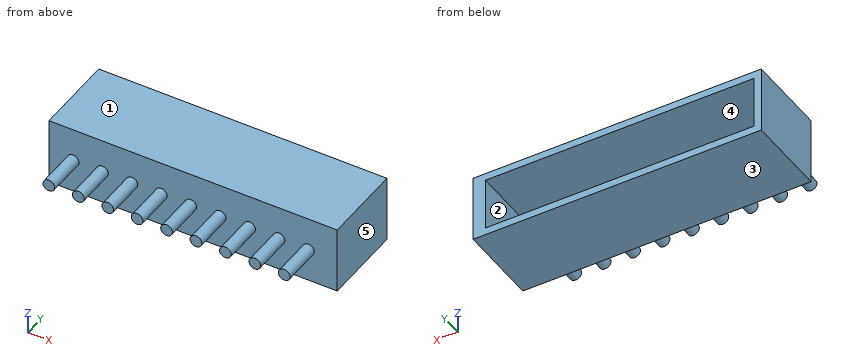
from build123d import *

# Parameters (mm, degrees)
F0_W     = 24.5
F0_H     = 5.7
F1_DEPTH = 7
F2_R     = 0.5
F3_DEPTH = 3.4
F4_W     = 22.82576
F4_H     = 4.464458
F5_DEPTH = 6.35


with BuildPart() as f1:
    # F0 (on Front) → F1 (new body)
    with BuildSketch(Plane.XZ):
        Rectangle(F0_W, F0_H)
    extrude(amount=F1_DEPTH)

    # F2 (on face) → F3 (join)
    with BuildSketch(Plane.XZ.offset(7)):
        with Locations((9.8, 0)):
            Circle(F2_R)
        with Locations((7.3, 0)):
            Circle(F2_R)
        with Locations((4.8, 0)):
            Circle(F2_R)
        with Locations((2.3, 0)):
            Circle(F2_R)
        with Locations((-0.2, 0)):
            Circle(F2_R)
        with Locations((-2.7, 0)):
            Circle(F2_R)
        with Locations((-5.2, 0)):
            Circle(F2_R)
        with Locations((-7.7, 0)):
            Circle(F2_R)
        with Locations((-10.2, 0)):
            Circle(F2_R)
    extrude(amount=F3_DEPTH)

    # F4 (on face) → F5 (cut)
    with BuildSketch(Plane(origin=(0, 0, 0), x_dir=(-1, 0, 0), z_dir=(0, 1, 0))):
        with Locations((0.214789, 0)):
            Rectangle(F4_W, F4_H)
    extrude(amount=-F5_DEPTH, mode=Mode.SUBTRACT)


solid = f1.part
Design review of the part built by this model. Coordinates are the model's own, in mm. Face numbers are marked on the shaded views. A direction names the side the tool comes from. Round coordinates to 2 decimals unless told otherwise and drop trailing zeros. Write each loop counter-clockwise with the first axis right and the second up, starting at its lowest first coordinate (ties: lowest second). Pieces come first, ordered by that corner, then holes. Notation, with made-up numbers: (-35.75, 84) - (-29.75, 84) arc R15 cw to (-29.75, 94) - close; hole circle Ø3 at (32.25, 27.25). An arc over 180 degrees is marked (long way). Return JSON: item names as keys, results as strings. Group by question number.
Item 1: We need section A-A on y = -9.5. Give the number of separate pieces and of enclosed holes in the cut face, and give its area (3 significant figures).
Item 2: Machinability: for the marked faces 1 and 2, which of the approach directions +Z, -Z, +X, -X, +Y, -Y give a long, thin tool a straight path to every point of the face, cutting with its end or side? Answer none if there is none.
Item 3: For probe 1 along X at (y, z) = (-5.75, 1.35); probe 2 along Z at (x, y) = (10.25, -5.75); probe 3 along Y at (x, z) = (-6, -1.8), list the stretches that pass through material, from the lowest coordinate up. Write a range as [from, to].
Item 4: The part is to be moulded in two halves that separate along X. For the marked faces 3, 4 and 5, say which applies: pulls with the +X half, pulls with the -X half, needs draft (parallel to the pull), parting line crosses it, or undercut.
Item 5: We need section D-D on z = -0.8. Write out the cut boundary in (x, y), and give its area (3 significant figures).
Item 6: We need section B-B on y = -4.5. Write out the cut boundary in (x, z).
Item 7: We need section C-C on x = 4.8. Write out the cut boundary in (y, z).
Model answer:
{
 "1": {"separate pieces": "9", "enclosed holes": "0", "area": "7.07 mm²"},
 "2": {"face 1": "+Z, +X, -X, +Y, -Y", "face 2": "+Y"},
 "3": {"probe 1": "x = [-12.25, -11.63], [11.2, 12.25]", "probe 2": "z = [-2.85, -2.23], [2.23, 2.85]", "probe 3": "y = [-7, -6.35]"},
 "4": {"face 3": "needs draft", "face 4": "undercut", "face 5": "pulls with the +X half"},
 "5": {"outline": "(-12.25, -7) - (12.25, -7) - (12.25, 0) - (11.2, 0) - (11.2, -6.35) - (-11.63, -6.35) - (-11.63, 0) - (-12.25, 0) - close", "area": "26.6 mm²"},
 "6": {"outline": "(-12.25, -2.85) - (12.25, -2.85) - (12.25, 2.85) - (-12.25, 2.85) - close; hole (-11.63, -2.23) - (11.2, -2.23) - (11.2, 2.23) - (-11.63, 2.23) - close"},
 "7": {"outline": "(-10.4, -0.5) - (-7, -0.5) - (-7, -2.85) - (0, -2.85) - (0, -2.23) - (-6.35, -2.23) - (-6.35, 2.23) - (0, 2.23) - (0, 2.85) - (-7, 2.85) - (-7, 0.5) - (-10.4, 0.5) - close"}
}
